```python
from build123d import *

# Parameters (mm, degrees)
PAD016_DEPTH            = 100
PAD019_DEPTH            = 10
SKETCH047_R             = 1.6
POCKET031_DEPTH         = 5
SKETCH048_R             = 3.5
POCKET027_DEPTH         = 1
SKETCH049_R             = 1.75
POCKET028_DEPTH         = 5
SKETCH050_R             = 3.5
POCKET029_DEPTH         = 1
PAD017_DEPTH            = 40
PAD018_DEPTH            = 3
SKETCH043_R             = 1.75
POCKET030_DEPTH         = 5
SKETCH054_R             = 3.5
POCKET034_DEPTH         = 1
SKETCH052_R             = 1.75
POCKET032_DEPTH         = 5
SKETCH053_R             = 3.5
POCKET033_DEPTH         = 1
BODY006_PLACEMENT_ANGLE = 180


with BuildPart() as part:
    # Sketch044 → Pad016 (new body)
    with BuildSketch(Plane.XY):
        Polygon((-53, -35), (-53, -53), (-35, -53), (-35, -48), (-48, -48), (-48, -35), align=None)
    extrude(amount=PAD016_DEPTH)

    # Sketch046 (on Face8 of Pad016) → Pad019 (join)
    with BuildSketch(Plane.XY.offset(100)):
        Polygon((-53, -35), (-53, -53), (-35, -53), (-35, -50), (-50, -50), (-50, -35), align=None)
    extrude(amount=PAD019_DEPTH)

    # Sketch047 (on Face14 of Pad019) → Pocket031 (cut)
    with BuildSketch(Plane.XZ.offset(53)):
        with Locations((-43, 105)):
            Circle(SKETCH047_R)
    extrude(amount=-POCKET031_DEPTH, mode=Mode.SUBTRACT)

    # Sketch048 (on Face14 of Pocket031) → Pocket027 (cut)
    with BuildSketch(Plane.XZ.offset(53)):
        with Locations((-43, 105)):
            Circle(SKETCH048_R)
    extrude(amount=-POCKET027_DEPTH, mode=Mode.SUBTRACT)

    # Sketch049 (on Face9 of Pocket027) → Pocket028 (cut)
    with BuildSketch(Plane(origin=(-53, 0, 0), x_dir=(0, -1, 0), z_dir=(-1, 0, 0))):
        with Locations((43, 105)):
            Circle(SKETCH049_R)
    extrude(amount=-POCKET028_DEPTH, mode=Mode.SUBTRACT)

    # Sketch050 (on Face9 of Pocket028) → Pocket029 (cut)
    with BuildSketch(Plane(origin=(-53, 0, 0), x_dir=(0, -1, 0), z_dir=(-1, 0, 0))):
        with Locations((43, 105)):
            Circle(SKETCH050_R)
    extrude(amount=-POCKET029_DEPTH, mode=Mode.SUBTRACT)

    # Sketch045 (on Face4 of Pocket029) → Pad017 (join)
    with BuildSketch(Plane(origin=(0, 0, 0), x_dir=(1, 0, 0), z_dir=(0, 0, -1))):
        Polygon((-35, 53), (-53, 53), (-53, 35), (-50, 35), (-50, 50), (-35, 50), align=None)
    extrude(amount=PAD017_DEPTH)

    # Sketch051 (on Face15 of Pad017) → Pad018 (join)
    with BuildSketch(Plane(origin=(0, 0, -40), x_dir=(1, 0, 0), z_dir=(0, 0, -1))):
        Polygon((-35, 50), (-35, 53), (-53, 53), (-53, 35), (-50, 35), align=None)
    extrude(amount=PAD018_DEPTH)

    # Sketch043 (on Face10 of Pad018) → Pocket030 (cut)
    with BuildSketch(Plane(origin=(-53, 0, 0), x_dir=(0, -1, 0), z_dir=(-1, 0, 0))):
        with Locations((43, -5)):
            Circle(SKETCH043_R)
    extrude(amount=-POCKET030_DEPTH, mode=Mode.SUBTRACT)

    # Sketch054 (on Face10 of Pocket030) → Pocket034 (cut)
    with BuildSketch(Plane(origin=(-53, 0, 0), x_dir=(0, -1, 0), z_dir=(-1, 0, 0))):
        with Locations((43, -5)):
            Circle(SKETCH054_R)
    extrude(amount=-POCKET034_DEPTH, mode=Mode.SUBTRACT)

    # Sketch052 (on Face19 of Pocket034) → Pocket032 (cut)
    with BuildSketch(Plane.XZ.offset(53)):
        with Locations((-43, -5)):
            Circle(SKETCH052_R)
    extrude(amount=-POCKET032_DEPTH, mode=Mode.SUBTRACT)

    # Sketch053 (on Face19 of Pocket032) → Pocket033 (cut)
    with BuildSketch(Plane.XZ.offset(53)):
        with Locations((-43, -5)):
            Circle(SKETCH053_R)
    extrude(amount=-POCKET033_DEPTH, mode=Mode.SUBTRACT)


with BuildPart() as part_1:
    # Body006 placement: moved
    add(part.part.rotate(Axis((0, 0, 0), (0, 0, 1)), BODY006_PLACEMENT_ANGLE))


solid = part_1.part
```
CAD build for the part. Positions are in the model's coordinates, mm. A direction names the side the tool comes from. Coordinates: 2 decimals unless noted, no trailing zeros. Loops run counter-clockwise (first coordinate to the right, second up) from the corner with the lowest first, then second, coordinate; pieces in that order, holes last. Notation, with made-up numbers: (-21, -27) - (35, -27) arc R6 cw to (35, -19) - close; hole circle Ø8 at (54, 8.25). An arc over 180 degrees is marked (long way). Return JSON: item names as keys, results as strings.
1. Mould opens along Y. For faces 5 (the cylindrical face through (51.014, 44.617, -5.67)), 6 (the flat face through (43, 42, -41)), 7 (the cylindrical face through (45.8, 52.5, 102.9)) say: released by +Y, released by -Y, zero draft, split by the parting line, or undercut.
Result:
{"face 5": "undercut", "face 6": "released by -Y", "face 7": "zero draft"}
2. Drop flat-ended pins along their axis: pin 1 (4 mm diameter, centred on y = 43, z = -5, fed in from -X); pin 2 (4 mm diameter, centred on x = 44, z = 68.5, fed in from -Y); pin 3 (2.5 mm diameter, centred on x = 43, z = 105, fed in from +Y); pin 4 (4.5 mm diameter, centred on x = 42, y = 44, fed in from +Z). Give the stop position or say it passes through.
Result:
{"pin 1": "stops at x = 50", "pin 2": "stops at y = 48", "pin 3": "passes through", "pin 4": "stops at z = -40"}
3. Band-saw the part on A-A (z = 105). Give the cut face in (x, y), and give its area (3 significant figures).
Result:
{"outline": "(35, 50) - (41.4, 50) - (41.4, 52) - (39.5, 52) - (39.5, 53) - (35, 53) - close; (44.6, 50) - (50, 50) - (50, 44.75) - (52, 44.75) - (52, 46.5) - (53, 46.5) - (53, 53) - (46.5, 53) - (46.5, 52) - (44.6, 52) - close; (50, 35) - (53, 35) - (53, 39.5) - (52, 39.5) - (52, 41.25) - (50, 41.25) - close", "area": "71.6 mm2"}
4. 3-axis set-ups, long thin cutter, end or side, ignore diameter. For faces 1 (the cylindrical face through (52.5, 40.2, 102.9)), 2 (the flat face through (45, 52, -6)), 3 (the flat face through (43, 50, -20)), 4 (the flat face through (41, 50, 105)): which of +Z, -Z, +X, -X, +Y, -Y reach the whole face in a straight line?
Result:
{"face 1": "+X", "face 2": "+Y", "face 3": "-X, -Y", "face 4": "+Z, -X, -Y"}
5. Band-saw the part on B-B (x = 43). Give the cut face in (y, z), and give its area (3 significant figures).
Result:
{"outline": "(42, -43) - (53, -43) - (53, -8.5) - (52, -8.5) - (52, -6.75) - (50, -6.75) - (50, -40) - (42, -40) - close; (48, 0) - (50, 0) - (50, -3.25) - (52, -3.25) - (52, -1.5) - (53, -1.5) - (53, 101.5) - (52, 101.5) - (52, 103.4) - (50, 103.4) - (50, 100) - (48, 100) - close; (50, 106.6) - (52, 106.6) - (52, 108.5) - (53, 108.5) - (53, 110) - (50, 110) - close", "area": "656 mm2"}
6. Probe L1, parallel to Z at x = 51.5, y = 43; L2, parallel to Z at x = 43, y = 52.4; L3, parallel to Y at x = 51.1, z = 105. List the from-to ranges inside material, lowest first. Write a range as from..to.
Result:
{"L1": "z = -43..-6.75, -3.25..103.25, 106.75..110", "L2": "z = -43..-8.5, -1.5..101.5, 108.5..110", "L3": "y = 35..41.25, 44.75..53"}
7. Band-saw the part on C-C (y = 36.5). Give the cut face in (x, z).
Result:
{"outline": "(48, 0) - (50, 0) - (50, -40) - (48.5, -40) - (48.5, -43) - (53, -43) - (53, 110) - (50, 110) - (50, 100) - (48, 100) - close"}
8. Band-saw the part on D-D (y = 42.5). Give the cut face in (x, z).
Result:
{"outline": "(42.5, -43) - (53, -43) - (53, -8.46) - (52, -8.46) - (52, -6.68) - (50, -6.68) - (50, -40) - (42.5, -40) - close; (48, 0) - (50, 0) - (50, -3.32) - (52, -3.32) - (52, -1.54) - (53, -1.54) - (53, 101.54) - (52, 101.54) - (52, 103.32) - (50, 103.32) - (50, 100) - (48, 100) - close; (50, 106.68) - (52, 106.68) - (52, 108.46) - (53, 108.46) - (53, 110) - (50, 110) - close"}
